Verification items for the finished model (mm, model axes). A direction names the side the tool comes from. Give positions to 0.01 mm unless a question says otherwise; leave off trailing zeros. Loops run counter-clockwise (first coordinate to the right, second up) from the corner with the lowest first, then second, coordinate; pieces in that order, holes last. Notation, with made-up numbers: (-6.5, 42.25) - (46.5, 42.25) arc R29 cw to (46.5, 62.25) - close; hole circle Ø10 at (88, 56.5). An arc over 180 degrees is marked (long way). Answer in a Markdown table with one row per item.
```python
from build123d import *

# Parameters (mm, degrees)
BOSS_EXTRUDE1_DEPTH      = 57.5
FILLET1_R                = 5
BOSS_EXTRUDE2_DEPTH      = 3.8
BOSS_EXTRUDE3_DEPTH      = 8.1
BOSS_EXTRUDE3_DEPTH_BACK = 11.9
SKETCH3_R                = 7.5
HOLE1_D                  = 7.5
BOSS_EXTRUDE4_DEPTH      = 8.1
BOSS_EXTRUDE4_DEPTH_BACK = 11.9
SKETCH7_W                = 3
SKETCH7_H                = 18.938620175
BOSS_EXTRUDE5_DEPTH      = 3
HOLE2_D                  = 3.8
HOLE2_DEPTH              = 4
FILLET2_R                = 2
HOLE3_D                  = 1.9
LPATTERN1_COUNT          = 2
LPATTERN1_PITCH          = 38


with BuildPart() as part:
    # Sketch1 → Boss-Extrude1 (new body)
    with BuildSketch(Plane(origin=(0, 0, 0), x_dir=(0, 0, -1), z_dir=(1, 0, 0))):
        Polygon((0, 5), (0, 10), (7, 10), (7, 7.5), (13.3, 7.5), (13.3, 10), (28.8, 10), (28.8, 0), (23.8, 0), (23.8, 5), align=None)
    extrude(amount=BOSS_EXTRUDE1_DEPTH)

    # Fillet1
    fillet1_edges = [part.edges().sort_by_distance(p)[0] for p in [
        (28.75, 0, -28.8),
    ]]
    fillet(fillet1_edges, radius=FILLET1_R - 0.0001)  # a hair under: the kernel refuses the full size

    # Sketch2 → Boss-Extrude2 (add)
    with BuildSketch(Plane(origin=(0, 0, -28.8), x_dir=(-1, 0, 0), z_dir=(0, 0, -1))):
        Polygon((-53.7, 10), (0, 10), (0, 19.6), (-38.105117767, 41.6), align=None)
    extrude(amount=-BOSS_EXTRUDE2_DEPTH)

    # Sketch3 → Boss-Extrude3 (add, two sides: drawn at the far end of the back side and taken through both)
    with BuildSketch(Plane.XY.offset(-25).offset(-BOSS_EXTRUDE3_DEPTH_BACK)):
        with Locations((13.7, 27.509698688)):
            Circle(SKETCH3_R)
    extrude(amount=BOSS_EXTRUDE3_DEPTH + BOSS_EXTRUDE3_DEPTH_BACK)

    # Hole1 (through all)
    with Locations(Plane.XY.offset(-16.9)):
        with Locations((13.7, 27.509698688)):
            Hole(HOLE1_D / 2)

    # Sketch6 → Boss-Extrude4 (add, two sides: drawn at the far end of the back side and taken through both)
    with BuildSketch(Plane.XY.offset(-25).offset(-BOSS_EXTRUDE4_DEPTH_BACK)):
        Polygon((38.105117767, 41.6), (41.692091359, 43.370203505), (50.073394311, 26.387120893), (46.486420719, 24.616917389), align=None)
    extrude(amount=BOSS_EXTRUDE4_DEPTH + BOSS_EXTRUDE4_DEPTH_BACK)

    # Sketch7 → Boss-Extrude5 (add)
    with BuildSketch(Plane(origin=(50.738305729, 25.039807043, 0), x_dir=(0, 0, -1), z_dir=(0.8967433980837525, 0.44255087616363914, 0))):
        with Locations((26.9, 10.971762018)):
            Rectangle(SKETCH7_W, SKETCH7_H)
    extrude(amount=BOSS_EXTRUDE5_DEPTH)

    # Hole2
    with Locations(Plane(origin=(50.738305729, 25.039807043, 0), x_dir=(0, 0, -1), z_dir=(0.8967433980837525, 0.44255087616363914, 0))):
        with Locations((34.4, 6.502451931), (22.4, 6.502451931), (22.4, 16.502451931), (34.4, 16.502451931)):
            Hole(HOLE2_D / 2, depth=HOLE2_DEPTH)

    # Fillet2
    fillet2_edges = [part.edges().sort_by_distance(p)[0] for p in [
        (39.898604563, 42.485101752, -36.9),
        (48.279907515, 25.502019141, -36.9),
        (48.279907515, 25.502019141, -16.9),
        (39.898604563, 42.485101752, -16.9),
    ]]
    fillet(fillet2_edges, radius=FILLET2_R)

    # Hole3 (through all)
    with Locations(Plane(origin=(0, 7.5, 0), x_dir=(1, 0, 0), z_dir=(0, 1, 0))):
        with Locations((10, 10)):
            hole3 = Hole(HOLE3_D / 2)

    # LPattern1: Hole3 ×2
    with Locations(*[(i * LPATTERN1_PITCH, 0, 0) for i in range(1, LPATTERN1_COUNT)]):
        add(hole3, mode=Mode.SUBTRACT)


solid = part.part
```
Q1. Tool access check on faces 1 (the face through (42.354, 32.99, -32.907)), 2 (the face through (45.824, 34.998, -21.21)), 3 (the face through (28, 9, -7)), 4 (the face through (48, 26, -17.5)). Record the directions out of +Z, -Z, +X, -X, +Y, -Y that give a thin tool (end or side, any length) a straight path to the whole face; none if there is none.
Completed:
| item | result |
|---|---|
| face 1 | -Z, -Y |
| face 2 | +Z, +X, +Y |
| face 3 | +X, -X, +Y |
| face 4 | +Z, +X |
Q2. Go/stop test with flat-tipped pins: P1, Ø8, axis at x = 42, y = 35, coming from the +Z side; P2, Ø1.5, axis at x = 23.5, z = -17.5, coming from the +Y side; P3, Ø4, axis at x = 42, y = 25, coming from the +Z side. Record where each tip stops, or that it passes through.
Completed:
| item | result |
|---|---|
| P1 | z = -16.9 |
| P2 | y = 10 |
| P3 | z = -25 |
Q3. Draft check along Y on faces 5 (the face through (10, 26, -16.9)), 6 (the face through (40.176, 41.986, -17.501)), 7 (the face through (40.78, 40.63, -22.65)). Enter one of: +Y half, -Y half, draft (parallel to the pull), parting line (faces both ways), or undercut.
Completed:
| item | result |
|---|---|
| face 5 | draft |
| face 6 | +Y half |
| face 7 | undercut |
Q4. Sectioned sample at A-A (z = -10). Record the cut outline in (x, y).
Completed:
| item | result |
|---|---|
| outline | (0, 5) - (9.05, 5) - (9.05, 7.5) - (0, 7.5) - close; (10.95, 5) - (47.05, 5) - (47.05, 7.5) - (10.95, 7.5) - close; (48.95, 5) - (57.5, 5) - (57.5, 7.5) - (48.95, 7.5) - close |
Q5. Thickness scan on line 1 (X direction, y = 7, z = -10); line 2 (Z direction, x = 46, y = 9.5); line 3 (Z direction, x = 48, y = 6.15). Record the ranges inside material, lowest first.
Completed:
| item | result |
|---|---|
| line 1 | 0 to 9.05, 10.95 to 47.05, 48.95 to 57.5 |
| line 2 | -28.8 to -13.3, -7 to 0 |
| line 3 | -28.8 to -10.95, -9.05 to 0 |
Q6. Sectioned sample at C-C (z = -31.5). Record the cut outline in (x, y), and give its area (3 significant figures).
Completed:
| item | result |
|---|---|
| outline | circle Ø15 at (13.7, 27.51); (38.11, 41.6) - (46.49, 24.62) - (50.07, 26.39) - (41.69, 43.37) - close; hole circle Ø7.5 at (13.7, 27.51) |
| area | 208 mm^2 |
